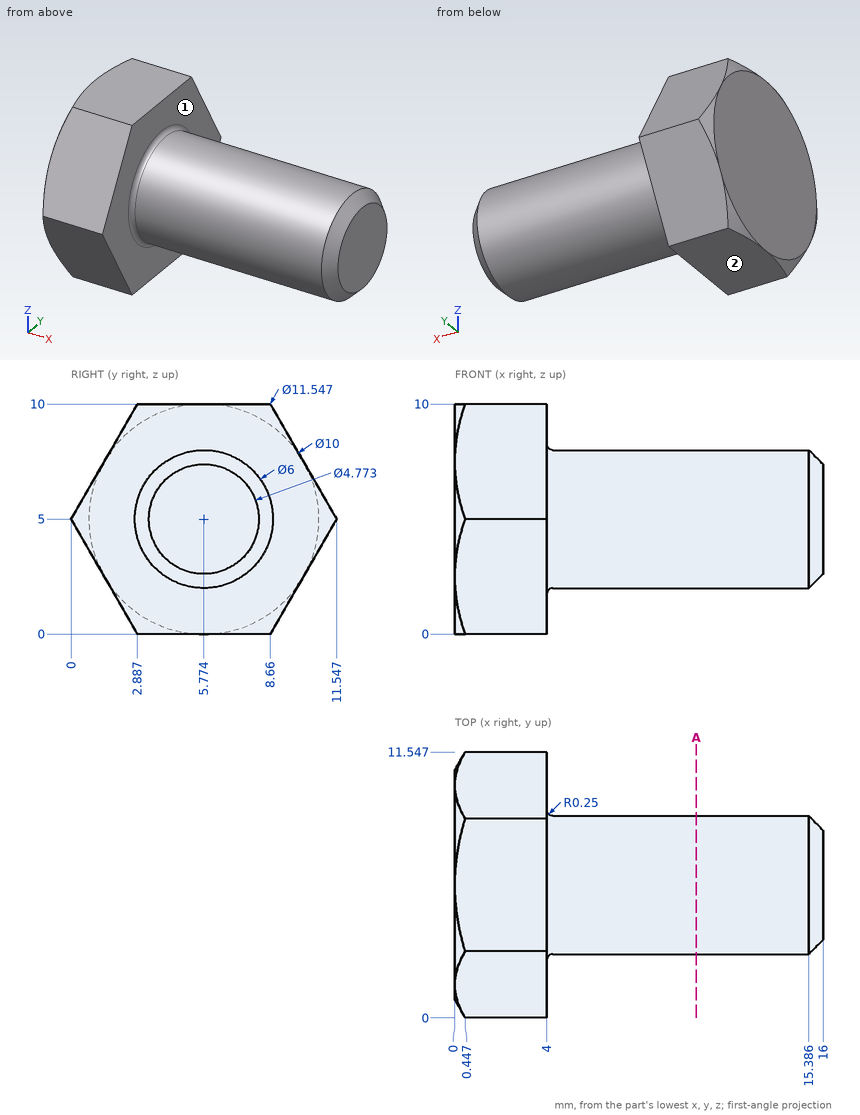
Study the drawing (mm; zero at the part's minimum x, y, z) and answer. A direction names the side the tool comes from. Give positions to 0.01 mm unless a question says otherwise; leave off trailing zeros. Order: outer loops, then holes, each group sorted by start corner. A loop starts at its lowest first (then second) coordinate and runs counter-clockwise, first axis right, second up.
1. Section A-A, the plane x = 10.5 is taken. Determine the outline of the cut face in (y, z), and give its area (3 significant figures).
Result sheet:
outline: circle Ø6 at (5.77, 5)
area: 28.3 mm2
2. Each of these flat-tipped pins is pushed along its axis until it touches: P1, Ø4, axis at x = 13, z = 2, coming from the +Y side; P2, Ø4, axis at x = 8, z = 6, coming from the +Y side; P3, Ø1, axis at x = 5, y = 8.5, coming from the -Z side. Where does it stop, or does it pass through?
Result sheet:
P1: stops at y = 8.6
P2: stops at y = 8.77
P3: stops at z = 2.99
3. Straight lines are drawn through the part: L1, parallel to X at y = 10, z = 6.25; L2, parallel to Z at x = 8.75, y = 6.5; L3, parallel to Y at x = 13.25, z = 6.5 (1 decimal). For each, find the intervals that lie inside material, in ascending order.
Result sheet:
L1: x = 0 to 4
L2: z = 2.09 to 7.91
L3: y = 3.2 to 8.4
4. For the marked faces 1 and 2, determine the directions among +Z, -Z, +X, -X, +Y, -Y from which every point of the face is accessible in a straight line to the end or side of a thin tool.
Result sheet:
face 1: +X
face 2: -Z, +X, -X, +Y, -Y
